```python
from build123d import *

# Parameters (mm, degrees)
CHAMFER1_SIZE   = 0.2032
CHAMFER2_SIZE   = 0.2032
LPATTERN1_COUNT = 3
LPATTERN1_PITCH = 2.286


with BuildPart() as part:
    # Sketch1 → Revolve1 (revolve)
    with BuildSketch(Plane.XY, mode=Mode.PRIVATE) as revolve1_sk:
        Polygon((0, 2.38125), (8.636, 2.38125), (8.636, 3.0734), (1.143, 3.0734), (1.143, 2.8194), (0.508, 2.8194), (0.508, 3.429), (0, 3.429), align=None)
    revolve(revolve1_sk.sketch.rotate(Axis((0, 0, 0), (-1, 0, 0)), 90), axis=Axis((0, 0, 0), (-1, 0, 0)))

    # Chamfer1
    chamfer1_edges = [part.edges().sort_by_distance(p)[0] for p in [
        (0, 0, 2.38125),
        (8.636, 0, 2.38125),
    ]]
    chamfer(chamfer1_edges, length=CHAMFER1_SIZE)

    # Chamfer2
    chamfer2_edges = [part.edges().sort_by_distance(p)[0] for p in [
        (8.636, 0, 3.0734),
    ]]
    chamfer(chamfer2_edges, length=CHAMFER2_SIZE)

    # Sketch2 → Cut-Revolve1 (revolve, cut)
    with BuildSketch(Plane.XY, mode=Mode.PRIVATE) as cut_revolve1_sk:
        Polygon((1.262276686, 3.360523314), (1.778, 2.8448), (2.293723314, 3.360523314), align=None)
    cut_revolve1 = revolve(cut_revolve1_sk.sketch.rotate(Axis((0, 0, 0), (-1, 0, 0)), 90), axis=Axis((0, 0, 0), (-1, 0, 0)), mode=Mode.SUBTRACT)

    # LPattern1: Cut-Revolve1 ×3
    with Locations(*[(i * LPATTERN1_PITCH, 0, 0) for i in range(1, LPATTERN1_COUNT)]):
        add(cut_revolve1, mode=Mode.SUBTRACT)


solid = part.part
```
Read the model definition and answer for the solid it produces. Units are mm, in the model's axes. A direction names the side the tool comes from. Give positions to 0.01 mm unless a question says otherwise; leave off trailing zeros. Write each loop counter-clockwise with the first axis right and the second up, starting at its lowest first coordinate (ties: lowest second). Pieces come first, ordered by that corner, then holes. Notation, with made-up numbers: (46, 28.5) - (90, 28.5) arc R12 ccw to (90, 49.5) - close; hole circle Ø9 at (-33.75, 59). An arc over 180 degrees is marked (long way). Write item = value, one per line. Start each with the question number.
Item 1: Find section A-A (x = 0.75). Give the vertices of the cut face in (y, z), then the cut area to 3 significant figures.
Item 2: Find the intervals of material crossed by probe 1 along Y at (x, z) = (4.75, 0); probe 2 along Y at (x, z) = (6, 1.75); probe 3 along Z at (x, y) = (3.25, 0.5), in increasing order. Write a range as [from, to].
Item 3: The mould has two halves that part along Z. Classify faces 1 (the cylindrical face through (5.194, -3.047, 0.4)), 2 (the flat face through (0.508, 3, -1)), 3 (the cylindrical face through (4.376, 2.325, 0.516)): +Z half, -Z half, draft (parallel to the pull), parting line (faces both ways), or undercut.
Item 4: Each of these flat-tipped pins is pushed along its axis until it touches: P1, Ø1, axis at x = 6, y = 1.5, coming from the -Z side; P2, Ø2, axis at x = 5.5, z = 2.5, coming from the +Y side; P3, Ø3, axis at x = 3.5, y = 1, coming from the +Z side. Where does it stop, or does it pass through?
Item 5: Find section B-B (x = 5.75). Give the vertices of the cut face in (y, z).
Item 6: A tool of negligible diameter and unlimited length cuts with its end or side. For faces 4 (the flat face through (0, -3, 0)), 5 (the cylindrical face through (1.343, -3.047, 0.4)), 6 (the cylindrical face through (0.821, 1.716, 2.237)), from which of +Z, -Z, +X, -X, +Y, -Y can it reach the whole face along a straight path? Write none if from no direction.
Response:
q1.outline = circle Ø5.64 at (0, 0); hole circle Ø4.76 at (0, 0)
q1.area = 7.16 mm²
q2.probe_1 = [-3.07, -2.38], [2.38, 3.07]
q2.probe_2 = [-2.53, -1.61], [1.61, 2.53]
q2.probe_3 = [-3.03, -2.33], [2.33, 3.03]
q3.face_1 = parting line
q3.face_2 = draft
q3.face_3 = undercut
q4.P1 = -2.91
q4.P2 = 2.68
q4.P3 = 3.07
q5.outline = circle Ø6.15 at (0, 0); hole circle Ø4.76 at (0, 0)
q6.face_4 = +Z, -Z, -X, +Y, -Y
q6.face_5 = +X
q6.face_6 = none
